Could you check a few things on this drawing? It's one solid part, dimensions in mm from its lowest x, y, z. A direction names the side the tool comes from. Give positions to 0.01 mm unless a question says otherwise; leave off trailing zeros. Order: outer loops, then holes, each group sorted by start corner. A loop starts at its lowest first (then second) coordinate and runs counter-clockwise, first axis right, second up. Notation, with made-up numbers: M 31.5,68 L 66.5,68 A28 ccw 66.5,96 Z; hole C 22,-21 d6. An arc over 180 degrees is marked long. One line per item, written item: value. Start each with the question number.
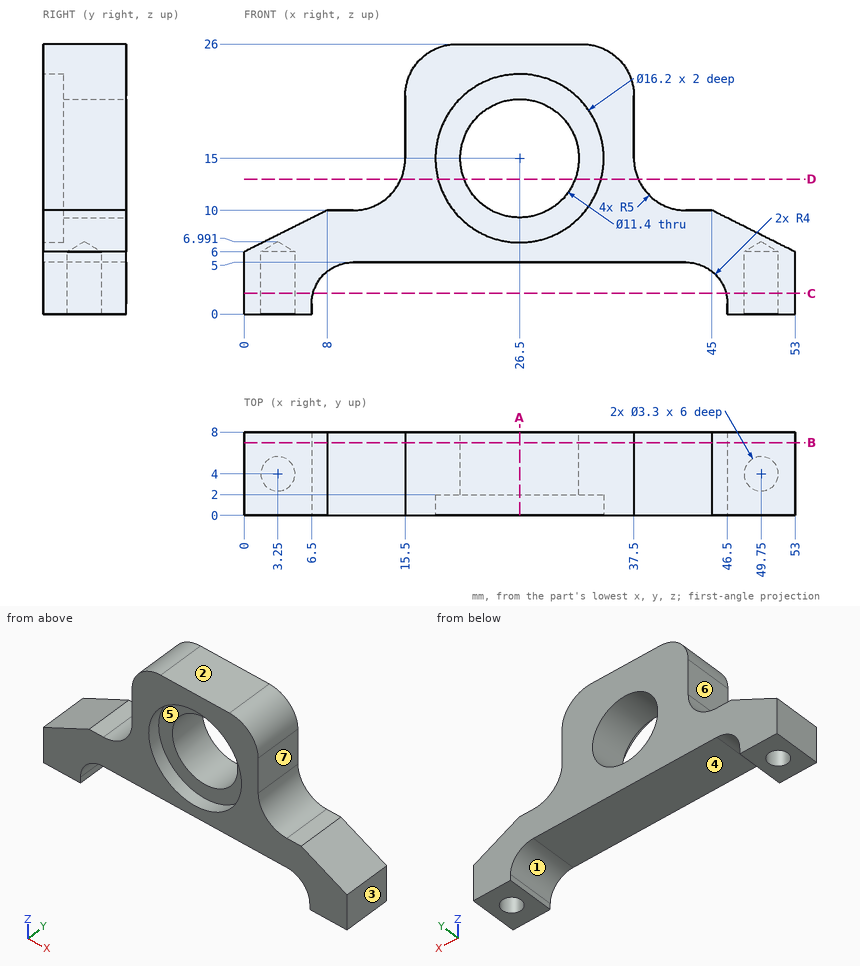
Item 1: I want a section at B-B on y = 7. Write out the boundary of the cut face in (x, z), plus the area to 3 significant figures.
Item 2: For the marked faces 4, 5, 6 and 7, which set-ups out of +Z, -Z, +X, -X, +Y, -Y let a thin tool reach every point of the face, with its end or its side?
Item 3: We'd pull the mould along X, two halves only. Please class the marked faces 1, 2 and 3: +X half, -X half, draft (parallel to the pull), parting line (faces both ways), or undercut.
Item 4: I want a section at A-A on x = 26.5. Write out the boundary of the cut face in (y, z), plus the area to 3 significant figures.
Item 5: I want a section at C-C on z = 2. Write out the boundary of the cut face in (x, y).
Item 6: Please list where these lines run through material, in increasing order: probe 1 along Z at (x, y) = (26.5, 4.8); probe 2 along Y at (x, z) = (49.75, 1.6); probe 3 along X at (y, z) = (3.25, 15.25) (1 decimal). Write a range as [from, to].
Item 7: Will these pins go through, and if not, where does the flat tip stop? P1, Ø14.5, axis at x = 26.5, z = 15, coming from the +Y side; P2, Ø2, axis at y = 3.5, z = 18, coming from the +X side; P3, Ø3, axis at x = 43.5, y = 5.5, coming from the +Z side (1 decimal); P4, Ø3, axis at y = 4, z = 15.5, coming from the +X side.
Item 8: I want a section at D-D on z = 13. Write out the boundary of the cut face in (x, y).
Answer below:
1. outline: M 0,0 L 6.5,0 L 6.5,1 A4 cw 10.5,5 L 42.5,5 A4 cw 46.5,1 L 46.5,0 L 53,0 L 53,6 L 45,10 L 42.5,10 A5 cw 37.5,15 L 37.5,21 A5 ccw 32.5,26 L 20.5,26 A5 ccw 15.5,21 L 15.5,15 A5 cw 10.5,10 L 8,10 L 0,6 Z; hole C 26.5,15 d11.4
1. area: 555 mm²
2. face 4: -Z, +Y, -Y
2. face 5: -Y
2. face 6: +Z, -X, +Y, -Y
2. face 7: +Z, +X, +Y, -Y
3. face 1: undercut
3. face 2: draft
3. face 3: +X half
4. outline: M 0,5 L 8,5 L 8,9.3 L 2,9.3 L 2,6.9 L 0,6.9 Z; M 0,23.1 L 2,23.1 L 2,20.7 L 8,20.7 L 8,26 L 0,26 Z
4. area: 67.2 mm²
5. outline: M 0,0 L 6.63,0 L 6.63,8 L 0,8 Z; M 46.37,0 L 53,0 L 53,8 L 46.37,8 Z; hole C 3.25,4 d3.3; hole C 49.75,4 d3.3
6. probe 1: z = [5, 9.3], [20.7, 26]
6. probe 2: y = [0, 2.35], [5.65, 8]
6. probe 3: x = [15.5, 20.8], [32.2, 37.5]
7. P1: stops at y = 8
7. P2: stops at x = 37.5
7. P3: stops at z = 10
7. P4: stops at x = 37.6
8. outline: M 15.08,0 L 18.65,0 L 18.65,2 L 21.16,2 L 21.16,8 L 15.08,8 Z; M 31.84,2 L 34.35,2 L 34.35,0 L 37.92,0 L 37.92,8 L 31.84,8 Z
